```python
from build123d import *

# Parameters (mm, degrees)
SKETCH_5_W          = 120
SKETCH_5_H          = 120
EXTRUDE_2_DEPTH     = 7
SKETCH_6_R          = 2.261709603
CUT_EXTRUDE_1_DEPTH = 7
SKETCH_9_R          = 4.406880206
CUT_EXTRUDE_2_DEPTH = 3
SKETCH_10_R         = 1.755844697
CUT_EXTRUDE_3_DEPTH = 7
SKETCH_11_R         = 2.744907592
CUT_EXTRUDE_4_DEPTH = 3


with BuildPart() as part:
    # 草图5 → 凸台-拉伸2 (new body)
    with BuildSketch(Plane.XY):
        with Locations((4.638432047, 17.423222422)):
            Rectangle(SKETCH_5_W, SKETCH_5_H)
    extrude(amount=EXTRUDE_2_DEPTH)

    # 草图6 → 切除-拉伸1 (cut)
    with BuildSketch(Plane.XY.offset(7)):
        with Locations((0, 72.710313561)):
            Circle(SKETCH_6_R)
    extrude(amount=-CUT_EXTRUDE_1_DEPTH, mode=Mode.SUBTRACT)

    # 草图9 → 切除-拉伸2 (cut)
    with BuildSketch(Plane.XY.offset(7)):
        with Locations((0, 72.710313561)):
            Circle(SKETCH_9_R)
    extrude(amount=-CUT_EXTRUDE_2_DEPTH, mode=Mode.SUBTRACT)

    # 草图10 → 切除-拉伸3 (cut)
    with BuildSketch(Plane.XY.offset(7)):
        with Locations((52.5, 26.710313561)):
            Circle(SKETCH_10_R)
    extrude(amount=-CUT_EXTRUDE_3_DEPTH, mode=Mode.SUBTRACT)

    # 草图11 → 切除-拉伸4 (cut)
    with BuildSketch(Plane.XY.offset(7)):
        with Locations((52.5, 26.710313561)):
            Circle(SKETCH_11_R)
    extrude(amount=-CUT_EXTRUDE_4_DEPTH, mode=Mode.SUBTRACT)


solid = part.part
```
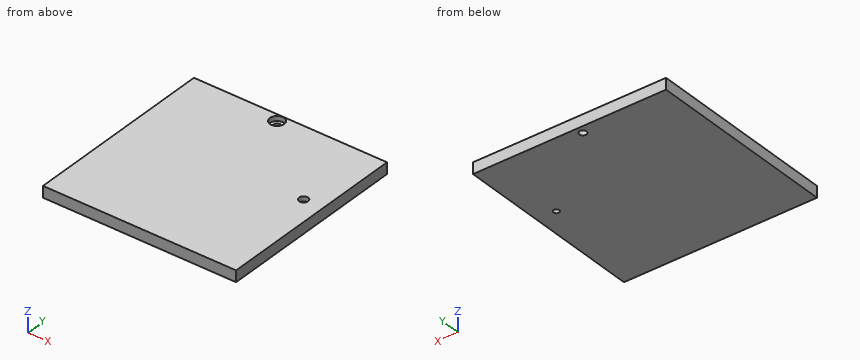
Geometry check sheet. Reference: the model listing, model coordinates, mm. Give positions to 0.01 mm unless a question says otherwise; leave off trailing zeros. Write each loop counter-clockwise with the first axis right and the second up, starting at its lowest first coordinate (ties: lowest second). Pieces come first, ordered by that corner, then holes.
1) Section check A-A, the plane x = 0. Record the boundary of the cut face in (y, z), and give its area (3 significant figures).
2) Section check B-B, the plane x = 52.5. Record the boundary of the cut face in (y, z), and give its area (3 significant figures).
3) Gauge pin test, flat ends, axial feed: pin 1 (7 mm diameter, centred on x = 0, y = 73.5, fed in from +Z); pin 2 (1.6 mm diameter, centred on x = 53, y = 27, fed in from +Z). Record the tip position at first contact, or that the pin passes through.
4) Material ranges on L1, parallel to Y at x = 52.5, z = 1.95; L2, parallel to Y at x = 0, z = 5.1; L3, parallel to X at y = 72, z = 0.5, recorded low to high.
Computed:
1. outline: (-42.58, 0) - (70.45, 0) - (70.45, 4) - (68.3, 4) - (68.3, 7) - (-42.58, 7) - close; (74.97, 0) - (77.42, 0) - (77.42, 7) - (77.12, 7) - (77.12, 4) - (74.97, 4) - close
1. area: 795 mm2
2. outline: (-42.58, 0) - (24.95, 0) - (24.95, 4) - (23.97, 4) - (23.97, 7) - (-42.58, 7) - close; (28.47, 0) - (77.42, 0) - (77.42, 7) - (29.46, 7) - (29.46, 4) - (28.47, 4) - close
2. area: 809 mm2
3. pin 1: stops at z = 4
3. pin 2: passes through
4. L1: y = -42.58 to 24.95, 28.47 to 77.42
4. L2: y = -42.58 to 68.3, 77.12 to 77.42
4. L3: x = -55.36 to -2.15, 2.15 to 64.64
